Geometry: final body of the model. Coordinates: model frame, mm. A direction names the side the tool comes from. Round coordinates to 2 decimals unless told otherwise and drop trailing zeros. Order: outer loops, then holes, each group sorted by start corner. A loop starts at its lowest first (then second) coordinate and runs counter-clockwise, first axis right, second up. Notation, with made-up numbers: (-12.75, -9.75) -> (0.25, -9.75) arc R30 cw to (0.25, 29.25) -> close; hole circle Ø3 at (46.5, 64.25). An arc over 180 degrees is marked (long way). Put each result on its own line as item: value.
```python
from build123d import *

# Parameters (mm, degrees)
SKETCH2_R                                  = 2
SKETCH2_R_2                                = 1.999999996
MAIN_FLOOR_EXTRUDE_DEPTH                   = 5
MAIN_FLOOR_CHAMFER_SIZE                    = 1
MOUNT_SCREW_COUNTERSINK_DEPTH              = 3
MOUNT_SCREW_COUNTERSINK_CHAMFER_SIZE       = 1
SKETCH6_R                                  = 2.05
BOTTOM_MOTOR_MOUNT_HOLES_DEPTH             = 183.816359737
SKETCH7_R                                  = 3.5
BOTTOM_MOTOR_MOUNT_HOLES_COUNTERSINK_DEPTH = 3


with BuildPart() as part:
    # Sketch2 → Main Floor Extrude (new body)
    with BuildSketch(Plane(origin=(0, 0, 0), x_dir=(1, 0, 0), z_dir=(0, 1, 0))):
        Polygon((129.222330464, 0), (129.222330464, -24.28090912), (82.337763357, -71.165476227), (89.511362957, -78.339075827), (91.560037368, -85.984832777), (85.984832777, -91.560037368), (78.339075822, -89.511362977), (71.165476214, -82.33776337), (24.280909108, -129.222330477), (0, -129.222330477), (-24.28090912, -129.222330477), (-71.165476227, -82.33776337), (-78.339075827, -89.51136297), (-85.984832777, -91.560037381), (-91.560037368, -85.984832789), (-89.511362977, -78.339075834), (-82.33776337, -71.165476227), (-129.222330477, -24.28090912), (-129.222330477, -1.3e-08), (-129.222330477, 24.280909108), (-82.33776337, 71.165476214), (-89.51136297, 78.339075814), (-91.560037381, 85.984832764), (-85.984832789, 91.560037355), (-78.339075834, 89.511362964), (-71.165476227, 82.337763357), (-24.28090912, 129.222330464), (-1.3e-08, 129.222330464), (24.280909108, 129.222330464), (71.165476214, 82.337763357), (78.339075814, 89.511362957), (85.984832764, 91.560037368), (91.560037355, 85.984832777), (89.511362964, 78.339075822), (82.337763357, 71.165476214), (129.222330464, 24.280909108), align=None)
        with Locations(Location((86.014718626, -86.014718626, 0), (0, 0, 270))):
            Circle(SKETCH2_R, mode=Mode.SUBTRACT)
        with Locations(Location((-86.014718626, -86.014718639, 0), (0, 0, 270))):
            Circle(SKETCH2_R, mode=Mode.SUBTRACT)
        with Locations(Location((-86.014718639, 86.014718613, 0), (0, 0, 270))):
            Circle(SKETCH2_R, mode=Mode.SUBTRACT)
        with Locations(Location((86.014718613, 86.014718626, 0), (0, 0, 270))):
            Circle(SKETCH2_R_2, mode=Mode.SUBTRACT)
    extrude(amount=MAIN_FLOOR_EXTRUDE_DEPTH)

    # Main Floor Chamfer
    main_floor_chamfer_edges = [part.edges().sort_by_distance(p)[0] for p in [
        (-74.752276027, 5, 85.92456317),
        (-47.723192674, 5, 105.780046923),
        (-6e-09, 5, 129.222330477),
        (47.723192661, 5, 105.780046923),
        (74.752276018, 5, 85.924563174),
        (82.161954299, 5, 90.535700173),
        (88.772435072, 5, 88.772435072),
        (85.924563161, 5, -74.752276018),
        (90.535700163, 5, 82.161954302),
        (85.924563157, 5, 74.752276027),
        (105.780046911, 5, 47.723192674),
        (90.53570016, 5, -82.161954299),
        (88.77243506, 5, -88.772435072),
        (82.161954289, 5, -90.535700163),
        (74.752276014, 5, -85.924563157),
        (47.723192661, 5, -105.780046911),
        (-6e-09, 5, -129.222330464),
        (-47.723192674, 5, -105.780046911),
        (-74.752276031, 5, -85.924563161),
        (129.222330464, 5, 6e-09),
        (-82.161954312, 5, -90.53570016),
        (-88.772435085, 5, -88.77243506),
        (-90.535700175, 5, -82.161954289),
        (-85.92456317, 5, -74.752276014),
        (-105.780046923, 5, -47.723192661),
        (-129.222330477, 5, 6e-09),
        (-105.780046923, 5, 47.723192674),
        (-85.924563174, 5, 74.752276031),
        (-90.535700173, 5, 82.161954312),
        (105.780046911, 5, -47.723192661),
        (-88.772435072, 5, 88.772435085),
        (-82.161954302, 5, 90.535700175),
    ]]
    chamfer(main_floor_chamfer_edges, length=MAIN_FLOOR_CHAMFER_SIZE)

    # Sketch3 → Mount Screw Countersink (cut)
    with BuildSketch(Plane(origin=(0, 0, 0), x_dir=(-1, 0, 0), z_dir=(0, -1, 0))):
        with BuildLine():
            Line((91.247308807, -86.297561351), (88.48959236, -83.539844904))
            ThreePointArc((88.48959236, -83.539844904), (83.539844892, -83.539844904), (83.539844892, -88.489592373))
            Line((83.539844892, -88.489592373), (86.297561338, -91.247308819))
            Line((86.297561338, -91.247308819), (91.247308807, -86.297561351))
        make_face()
        with BuildLine():
            Line((-86.297561351, -91.247308807), (-83.539844904, -88.48959236))
            ThreePointArc((-83.539844904, -88.48959236), (-83.539844904, -83.539844892), (-88.489592373, -83.539844892))
            Line((-88.489592373, -83.539844892), (-91.247308819, -86.297561338))
            Line((-91.247308819, -86.297561338), (-86.297561351, -91.247308807))
        make_face()
        with BuildLine():
            Line((-91.247308807, 86.297561351), (-88.48959236, 83.539844904))
            ThreePointArc((-88.48959236, 83.539844904), (-83.539844892, 83.539844904), (-83.539844892, 88.489592373))
            Line((-83.539844892, 88.489592373), (-86.297561338, 91.247308819))
            Line((-86.297561338, 91.247308819), (-91.247308807, 86.297561351))
        make_face()
        with BuildLine():
            Line((86.297561351, 91.247308807), (83.539844904, 88.48959236))
            ThreePointArc((83.539844904, 88.48959236), (83.539844904, 83.539844892), (88.489592373, 83.539844892))
            Line((88.489592373, 83.539844892), (91.247308819, 86.297561338))
            Line((91.247308819, 86.297561338), (86.297561351, 91.247308807))
        make_face()
    extrude(amount=-MOUNT_SCREW_COUNTERSINK_DEPTH, mode=Mode.SUBTRACT)

    # Mount Screw Countersink Chamfer
    mount_screw_countersink_chamfer_edges = [part.edges().sort_by_distance(p)[0] for p in [
        (-84.918703128, 0, -89.868450583),
        (-89.868450596, 0, -84.918703115),
        (-83.539844904, 0, -83.539844892),
        (89.868450583, 0, -84.918703128),
        (84.918703115, 0, -89.868450596),
        (83.539844892, 0, -83.539844904),
        (84.918703128, 0, 89.868450583),
        (89.868450596, 0, 84.918703115),
        (83.539844904, 0, 83.539844892),
        (-89.868450583, 0, 84.918703128),
        (-84.918703115, 0, 89.868450596),
        (-83.539844892, 0, 83.539844904),
    ]]
    chamfer(mount_screw_countersink_chamfer_edges, length=MOUNT_SCREW_COUNTERSINK_CHAMFER_SIZE)

    # Sketch6 → Bottom Motor Mount Holes (cut, through all)
    with BuildSketch(Plane(origin=(0, 5, 0), x_dir=(1, 0, 0), z_dir=(0, 1, 0))):
        with Locations(Location((-16, 16, 0), (0, 0, 270))):
            Circle(SKETCH6_R)
        with Locations(Location((16, 16, 0), (0, 0, 270))):
            Circle(SKETCH6_R)
        with Locations(Location((16, -16, 0), (0, 0, 270))):
            Circle(SKETCH6_R)
        with Locations(Location((-16, -16, 0), (0, 0, 270))):
            Circle(SKETCH6_R)
    extrude(amount=-BOTTOM_MOTOR_MOUNT_HOLES_DEPTH, mode=Mode.SUBTRACT)

    # Sketch7 → Bottom Motor Mount Holes Countersink (cut)
    with BuildSketch(Plane(origin=(0, 0, 0), x_dir=(-1, 0, 0), z_dir=(0, -1, 0))):
        with Locations(Location((16, -16, 0), (0, 0, 90))):
            Circle(SKETCH7_R)
        with Locations(Location((-16, -16, 0), (0, 0, 90))):
            Circle(SKETCH7_R)
        with Locations(Location((-16, 16, 0), (0, 0, 90))):
            Circle(SKETCH7_R)
        with Locations(Location((16, 16, 0), (0, 0, 90))):
            Circle(SKETCH7_R)
    extrude(amount=-BOTTOM_MOTOR_MOUNT_HOLES_COUNTERSINK_DEPTH, mode=Mode.SUBTRACT)


solid = part.part
```
1. Cut plane B-B on x = 36. Return loops of the section in (y, z).
Ans:
outline: (0, -117.5) -> (4, -117.5) -> (5, -116.09) -> (5, 116.09) -> (4, 117.5) -> (0, 117.5) -> close
2. Set-up query: faces 1 (the face through (-85.157, 4.507, -74.702)), 2 (the face through (-74.812, 4.507, -85.268)), 3 (the face through (-85.87, 1.97, -74.7)), 4 (the face through (-88, 3, 88)). Return all of +Z, -Z, +X, -X, +Y, -Y with unobstructed straight access to the full face (end or side cutting, diameter ignored); none if empty.
Ans:
face 1: -X, +Y
face 2: -Z, +Y
face 3: -X, +Y, -Y
face 4: -Y
3. Contact query for flat-ended pins moving along their axis: P1, Ø2.5, axis at x = 86.01, z = -86.01, coming from the -Y side; P2, Ø6.5, axis at x = -16, z = 16, coming from the -Y side; P3, Ø1.5, axis at y = 2.5, z = 53.5, coming from the +X side. Output: stop coordinate, or through.
Ans:
P1: through
P2: y = 3
P3: x = 100.75
4. Draft query along Z for faces 5 (the face through (48.1, 4.5, 104.7)), 6 (the face through (-83.49, 1.99, -83.59)), 7 (the face through (-48.051, 1.972, -105.452)), 8 (the face through (83.59, 1.99, -83.49)). Return one class per face: +Z half, -Z half, draft (parallel to the pull), parting line (faces both ways), or undercut.
Ans:
face 5: +Z half
face 6: undercut
face 7: -Z half
face 8: undercut
5. Material intervals for probe 1 along X at (y, z) = (3.5, -16); probe 2 along X at (y, z) = (1.1, 88); probe 3 along X at (y, z) = (2.45, -84), sorted ascending.
Ans:
probe 1: -129.22 to -18.05, -13.95 to 13.95, 18.05 to 129.22
probe 2: -83.13 to -76.83, -65.5 to 65.5, 76.83 to 83.13
probe 3: -91.03 to -88.95, -83.15 to -72.83, -69.5 to 69.5, 72.83 to 83.15, 88.95 to 91.03
6. Cut plane A-A on y = 2.1. State how many separate pieces and enclosed holes the cut face has, and give its area (3 significant figures).
Ans:
separate pieces: 1
enclosed holes: 4
area: 45,400 mm²
7. Cut plane C-C on z = 34. Return loops of the section in (x, y), and give its area (3 significant figures).
Ans:
outline: (-119.5, 0) -> (119.5, 0) -> (119.5, 4) -> (118.09, 5) -> (-118.09, 5) -> (-119.5, 4) -> close
area: 1,190 mm²
